Verification items for the finished model (mm, model axes). Round coordinates to 2 decimals unless told otherwise and drop trailing zeros. Write each loop counter-clockwise with the first axis right and the second up, starting at its lowest first coordinate (ties: lowest second). Pieces come first, ordered by that corner, then holes. Notation, with made-up numbers: (-21.5, 3.25) -> (24.5, 3.25) arc R23 cw to (24.5, 38.25) -> close; hole circle Ø5 at (-36.75, 56). An arc over 180 degrees is marked (long way). Answer as a JSON object with one key per item and string values. Group by question number.
(1) Sectioned sample at B-B on z = -5.5. Record the cut outline in (x, y), and give its area (3 significant figures).
(2) Gauge pin test, flat ends, axial feed: pin 1 Ø0.5 at (x, y) = (-32, 49.5) entering from -Z; pin 2 Ø1.5 at (y, z) = (36.5, 0) entering from +X; pin 3 Ø1.4 at (x, z) = (0, 0.5) entering from -Y. Record the tip position at first contact, or that the pin passes through.
(3) Sectioned sample at C-C on x = -4. Record the cut outline in (y, z).
(4) Scan lines: L1, parallel to Y at x = 69.25, z = 0; L2, parallel to Z at x = -3.5, y = 3.5; L3, parallel to Y at x = 9, z = -1. Record each from-to range of solid material in increasing order. Write a range as from..to.
(5) Sectioned sample at A-A on y = 6. Record the cut outline in (x, z) (3 decimals), and give its area (3 significant figures).
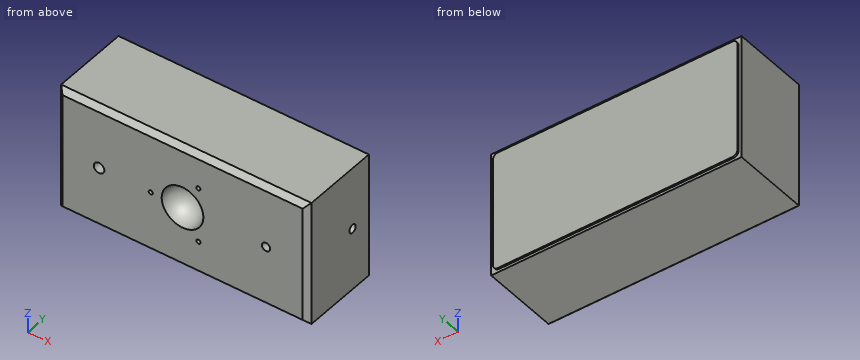
```python
from build123d import *

# Parameters (mm, degrees)
SKETCH1_W                          = 150
SKETCH1_H                          = 75
EXTRUDE1_DEPTH                     = 48.9966
CIRPATTERN1_COUNT                  = 3
M5X0_8_TAPPED_HOLE1_D              = 4.2
M5X0_8_TAPPED_HOLE1_DEPTH          = 15.24
M5X0_8_TAPPED_HOLE1_CBORE_D        = 5
M5X0_8_TAPPED_HOLE1_CBORE_DEPTH    = 10.16
M5X0_8_TAPPED_HOLE1_TIP            = 1.2618073
F_1_4_0_25_DIAMETER_HOLE1_D        = 6.35
F_1_4_0_25_DIAMETER_HOLE1_DEPTH    = 9.652
F_1_4_0_25_DIAMETER_HOLE1_TIP      = 1.907732465
M5X0_8_TAPPED_HOLE2_D              = 4.2
M5X0_8_TAPPED_HOLE2_DEPTH          = 15.24
M5X0_8_TAPPED_HOLE2_CBORE_D        = 5
M5X0_8_TAPPED_HOLE2_CBORE_DEPTH    = 10.16
M5X0_8_TAPPED_HOLE2_TIP            = 1.2618073
F_3_16_0_1875_DIAMETER_HOLE1_D     = 4.7625
F_3_16_0_1875_DIAMETER_HOLE1_DEPTH = 12.446
CHAMFER1_SIZE                      = 3.048
EXTRUDE2_DEPTH                     = 0.96519992


with BuildPart() as part:
    # Sketch1 → Extrude1 (new body)
    with BuildSketch(Plane(origin=(0, 0, 0), x_dir=(1, 0, 0), z_dir=(0, 1, 0))):
        Rectangle(SKETCH1_W, SKETCH1_H)
    extrude(amount=EXTRUDE1_DEPTH)

    # Sketch3 → Cut-Revolve1 (revolve, cut)
    with BuildSketch(Plane.XY):
        with BuildLine():
            Line((0, -13.0148), (0, 11.9988))
            ThreePointArc((0, 11.9988), (-12.5068, -0.508), (0, -13.0148))
        make_face()
    revolve(axis=Axis((0, -13.0148, 0), (0, 1, 0)), mode=Mode.SUBTRACT)

    # Sketch4 → M3x0.5 Tapped Hole1 (revolve, cut)
    with BuildSketch(Plane(origin=(-19.05, 0, 0), x_dir=(0, 0, -1), z_dir=(1, 0, 0))):
        Polygon((0, 0), (0, 8.571684836), (1.25, 7.849997), (1.25, 0), align=None)
    m3x0_5_tapped_hole1 = revolve(axis=Axis((-19.05, -6.35, 0), (0, 1, 0)), mode=Mode.SUBTRACT)

    # CirPattern1: M3x0.5 Tapped Hole1 ×3 about axis
    cirpattern1_axis = Axis((0, 0, 0), (0, 1, 0))
    for i in range(1, CIRPATTERN1_COUNT):
        add(m3x0_5_tapped_hole1.rotate(cirpattern1_axis, i * 360 / CIRPATTERN1_COUNT), mode=Mode.SUBTRACT)

    # M5x0.8 Tapped Hole1
    with Locations(Plane(origin=(3.180539722, 0, -8.853139463), x_dir=(-1, 0, 0), z_dir=(0, -1, 0))):
        with Locations((-46.819460278, -8.853139463)):
            CounterBoreHole(M5X0_8_TAPPED_HOLE1_D / 2, M5X0_8_TAPPED_HOLE1_CBORE_D / 2, M5X0_8_TAPPED_HOLE1_CBORE_DEPTH, depth=M5X0_8_TAPPED_HOLE1_DEPTH)
            with Locations((0, 0, -(M5X0_8_TAPPED_HOLE1_DEPTH + M5X0_8_TAPPED_HOLE1_TIP / 2))):  # 118° drill point
                Cone(0, M5X0_8_TAPPED_HOLE1_D / 2, M5X0_8_TAPPED_HOLE1_TIP, mode=Mode.SUBTRACT)

    # 1_4 _0.25_ Diameter Hole1
    with Locations(Plane(origin=(7.783143684, 0, 5.786983083), x_dir=(-1, 0, 0), z_dir=(0, -1, 0))):
        with Locations((57.783143684, 5.786983083)):
            Hole(F_1_4_0_25_DIAMETER_HOLE1_D / 2, depth=F_1_4_0_25_DIAMETER_HOLE1_DEPTH)
            with Locations((0, 0, -(F_1_4_0_25_DIAMETER_HOLE1_DEPTH + F_1_4_0_25_DIAMETER_HOLE1_TIP / 2))):  # 118° drill point
                Cone(0, F_1_4_0_25_DIAMETER_HOLE1_D / 2, F_1_4_0_25_DIAMETER_HOLE1_TIP, mode=Mode.SUBTRACT)

    # M5x0.8 Tapped Hole2
    with Locations(Plane(origin=(75, -6.107751103, -10.810874371), x_dir=(0, 0, 1), z_dir=(1, 0, 0))):
        with Locations((10.810874371, -42.099551103)):
            CounterBoreHole(M5X0_8_TAPPED_HOLE2_D / 2, M5X0_8_TAPPED_HOLE2_CBORE_D / 2, M5X0_8_TAPPED_HOLE2_CBORE_DEPTH, depth=M5X0_8_TAPPED_HOLE2_DEPTH)
            with Locations((0, 0, -(M5X0_8_TAPPED_HOLE2_DEPTH + M5X0_8_TAPPED_HOLE2_TIP / 2))):  # 118° drill point
                Cone(0, M5X0_8_TAPPED_HOLE2_D / 2, M5X0_8_TAPPED_HOLE2_TIP, mode=Mode.SUBTRACT)

    # 3_16 _0.1875_ Diameter Hole1
    with Locations(Plane(origin=(-43.604904101, 0, -18.203855586), x_dir=(-1, 0, 0), z_dir=(0, -1, 0))):
        with Locations((-43.611104101, -18.188055586)):
            Hole(F_3_16_0_1875_DIAMETER_HOLE1_D / 2, depth=F_3_16_0_1875_DIAMETER_HOLE1_DEPTH)

    # Chamfer1
    chamfer1_edges = [part.edges().sort_by_distance(p)[0] for p in [
        (0, 0, -37.5),
        (75, 0, 0),
        (0, 0, 37.5),
        (-75, 0, 0),
    ]]
    chamfer(chamfer1_edges, length=CHAMFER1_SIZE)

    # Sketch14 → Extrude2 (add)
    with BuildSketch(Plane.XZ.offset(-48.9966)):
        with BuildLine():
            Line((70.1613, 35.7474), (-70.1991, 35.7474))
            ThreePointArc((-70.1991, 35.7474), (-72.381302237, 34.843502237), (-73.2852, 32.6613))
            Line((-73.2852, 32.6613), (-73.2852, -32.6929))
            ThreePointArc((-73.2852, -32.6929), (-72.381302237, -34.875102237), (-70.1991, -35.779))
            Line((-70.1991, -35.779), (70.1613, -35.779))
            ThreePointArc((70.1613, -35.779), (72.343502237, -34.875102237), (73.2474, -32.6929))
            Line((73.2474, -32.6929), (73.2474, 32.6613))
            ThreePointArc((73.2474, 32.6613), (72.343502237, 34.843502237), (70.1613, 35.7474))
        make_face()
    extrude(amount=-EXTRUDE2_DEPTH)


solid = part.part
```
Computed values:
{
 "1": {"outline": "(-75, 3.05) -> (-71.95, 0) -> (-11.22, 0) arc R11.23 cw to (11.22, 0) -> (71.95, 0) -> (75, 3.05) -> (75, 49) -> (73.25, 49) -> (73.25, 49.96) -> (-73.29, 49.96) -> (-73.29, 49) -> (-75, 49) -> close", "area": "7,290 mm2"},
 "2": {"pin 1": "z = -35.78", "pin 2": "x = 59.25", "pin 3": "y = 12.45"},
 "3": {"outline": "(0, -34.45) -> (3.05, -37.5) -> (49, -37.5) -> (49, -35.78) -> (49.96, -35.78) -> (49.96, 35.75) -> (49, 35.75) -> (49, 37.5) -> (3.05, 37.5) -> (0, 34.45) -> (0, 11.84) arc R11.85 cw to (0, -11.84) -> close"},
 "4": {"L1": "0..33.49, 38.49..49.96", "L2": "-37.5..-11.32, 11.32..37.5", "L3": "8.12..49.96"},
 "5": {"outline": "(-75, -37.5) -> (75, -37.5) -> (75, 37.5) -> (-75, 37.5) -> close; hole circle Ø6.35 at (-50, 0); hole circle Ø2.5 at (-19.05, 0); hole circle Ø21.36 at (0, 0); hole circle Ø2.5 at (9.525, -16.498); hole circle Ø2.5 at (9.525, 16.498); hole circle Ø5 at (50, 0)", "area": "10,800 mm2"}
}
